```python
from build123d import *

# Parameters (mm, degrees)
SKETCH2_W               = 3
SKETCH2_H               = 18.2
BOSS_EXTRUDE1_DEPTH     = 26
CIRPATTERN1_COUNT       = 6
CUT_EXTRUDE1_DEPTH      = 41.546269865
CUT_EXTRUDE1_DEPTH_BACK = 41.546269865
SKETCH3_W               = 4
SKETCH3_H               = 4
FILLET1_R               = 2


with BuildPart() as part:
    # Sketch1 → Revolve1 (revolve)
    with BuildSketch(Plane(origin=(0, 0, 0), x_dir=(0, 0, -1), z_dir=(1, 0, 0)), mode=Mode.PRIVATE) as revolve1_sk:
        Polygon((0, 22), (1.7, 22), (1.7, 20.2), (4.2, 20.2), (4.2, 22), (6.2, 22), (6.5, 20.2), (19.5, 20.2), (19.8, 22), (21.8, 22), (21.8, 20.2), (24.3, 20.2), (24.3, 22), (26, 22), (26, 18.2), (0, 18.2), align=None)
    revolve(revolve1_sk.sketch.rotate(Axis((0, 0, 0.322174052), (0, 0, -1)), 90), axis=Axis((0, 0, 0.322174052), (0, 0, -1)))

    # Sketch2 → Boss-Extrude1 (add)
    with BuildSketch(Plane.XY):
        with Locations((0, 9.1)):
            Rectangle(SKETCH2_W, SKETCH2_H)
    boss_extrude1 = extrude(amount=-BOSS_EXTRUDE1_DEPTH)

    # CirPattern1: Boss-Extrude1 ×6 about axis
    cirpattern1_axis = Axis((0, 0, 0), (0, 0, 1))
    for i in range(1, CIRPATTERN1_COUNT):
        add(boss_extrude1.rotate(cirpattern1_axis, i * 360 / CIRPATTERN1_COUNT))

    # Sketch3 → Cut-Extrude1 (cut, two sides: drawn at the far end of the back side and taken through both)
    with BuildSketch(Plane.XY.offset(-CUT_EXTRUDE1_DEPTH_BACK)):
        Rectangle(SKETCH3_W, SKETCH3_H)
    extrude(amount=CUT_EXTRUDE1_DEPTH + CUT_EXTRUDE1_DEPTH_BACK, mode=Mode.SUBTRACT)

    # Fillet1
    fillet1_edges = [part.edges().sort_by_distance(p)[0] for p in [
        (3, 0, -13),
        (1.5, -2.598076211, -13),
        (-1.5, -2.598076211, -13),
        (-3, 0, -13),
        (16.458039343, 7.770002637, -13),
        (14.958039343, 10.368078849, -13),
        (16.458039343, -7.770002637, -13),
        (14.958039343, -10.368078849, -13),
        (-14.958039343, 10.368078849, -13),
        (-1.5, -18.138081486, -13),
        (1.5, -18.138081486, -13),
        (-16.458039343, -7.770002637, -13),
        (-14.958039343, -10.368078849, -13),
        (-16.458039343, 7.770002637, -13),
        (1.5, 18.138081486, -13),
        (-1.5, 18.138081486, -13),
        (-1.5, 2.598076211, -13),
        (1.5, 2.598076211, -13),
    ]]
    fillet(fillet1_edges, radius=FILLET1_R)


solid = part.part
```
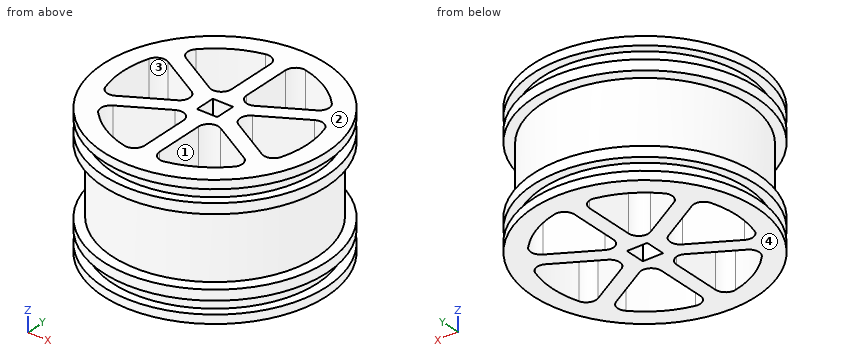
The listing builds one solid part. Answer for the finished solid, in the listing's coordinates (mm). Face numbers are marked on the shaded views. A direction names the side the tool comes from. Round coordinates to 2 decimals unless told otherwise and drop trailing zeros. Answer as a JSON object with one key per item and string values. Group by question number.
Q1. Section B-B (z = -4.75) is taken. Count the separate pieces of the cut face and the enclosed holes in it, plus the area to 3 significant figures.
Q2. Which of the six approach directions +Z, -Z, +X, -X, +Y, -Y give full straight-line access (tool end or side, diameter ignored) to the marked faces 3 and 4?
Q3. Straight lines are drawn through the part: line 1 along Y through (x, z) = (-7, -15.5); line 2 along X through (y, z) = (16.5, -18.25); line 3 along Y through (x, z) = (-4, -15.75) (3 decimals). For each, find the intervals that lie inside material, in ascending order.
Q4. Each of these flat-tipped pins is pushed along its axis until it touches: pin 1 Ø8 at (y, z) = (-13, -11) entering from +X; pin 2 Ø1 at (x, z) = (2.5, -9) entering from -Y; pin 3 Ø1.2 at (x, z) = (-0.5, -16) entering from +Y; pin 4 Ø2 at (x, y) = (8.5, 14) entering from -Z. Where does it stop, or does it pass through?
Q5. Determine the mould class of the marked faces 1 and 2 for opening direction Y: pulls with the +Y half, pulls with the -Y half, needs draft (parallel to the pull), parting line crosses it, or undercut.
Check values:
{
 "1": {"separate pieces": "1", "enclosed holes": "7", "area": "799 mm^2"},
 "2": {"face 3": "+Z, -Z", "face 4": "-Z, +X, -X, +Y, -Y"},
 "3": {"line 1": "-18.95 to -16.8, -5.77 to -2.31, 2.31 to 5.77, 16.8 to 18.95", "line 2": "-11.65 to -7.68, -1.62 to 1.62, 7.68 to 11.65", "line 3": "-19.8 to -17.755, -4.126 to 4.126, 17.755 to 19.8"},
 "4": {"pin 1": "x = 18.08", "pin 2": "y = -20.1", "pin 3": "y = 20.2", "pin 4": "through"},
 "5": {"face 1": "undercut", "face 2": "needs draft"}
}
